```python
from build123d import *

# Parameters (mm, degrees)
F2_R     = 254
F3_DEPTH = 635
F4_R     = 127
F5_DEPTH = 1270.001


with BuildPart() as f1:
    # F0 (on Front) → F1 (revolve)
    with BuildSketch(Plane.XZ):
        with BuildLine():
            Line((-330.2, 381), (-330.2, 254))
            Line((-330.2, 254), (330.2, 254))
            Line((330.2, 254), (330.2, 381))
            Line((330.2, 381), (203.2, 381))
            Line((203.2, 381), (203.2, 889))
            Line((203.2, 889), (152.4, 889))
            ThreePointArc((152.4, 889), (0, 736.6), (-152.4, 889))
            Line((-152.4, 889), (-203.2, 889))
            Line((-203.2, 889), (-203.2, 381))
            Line((-203.2, 381), (-330.2, 381))
        make_face()
    revolve(axis=Axis((165.1, 0, 0), (1, 0, 0)))

    # F2 (on Right) → F3 (join, symmetric)
    with BuildSketch(Plane.YZ):
        Circle(F2_R)
    extrude(amount=F3_DEPTH, both=True)

    # F4 (on face) → F5 (cut, through all)
    with BuildSketch(Plane.YZ.offset(635)):
        Circle(F4_R)
    extrude(amount=-F5_DEPTH, mode=Mode.SUBTRACT)


solid = f1.part
```
Read the model definition and answer for the solid it produces. Units are mm, in the model's axes. A direction names the side the tool comes from. Give positions to 0.01 mm unless a question says otherwise; leave off trailing zeros. Order: outer loops, then holes, each group sorted by start corner. A loop starts at its lowest first (then second) coordinate and runs counter-clockwise, first axis right, second up.
(1) Find section C-C (x = -179.5). Give the vertices of the cut face in (y, z), plus the area to 3 significant figures.
(2) Find section A-A (y = 0). Give the vertices of the cut face in (x, z).
(3) For faces 4 (the flat face through (203.2, -12, -383)), 5 (the flat face through (-203.2, -12, 383)), 6 (the flat face through (-635, 53, 116)), determine the directions among +Z, -Z, +X, -X, +Y, -Y from which every point of the face is accessible in a straight line to the end or side of a thin tool.
(4) Find section D-D (x = -422). Give the vertices of the cut face in (y, z), plus the area to 3 significant figures.
(5) Straight lines are drawn through the part: L1, parallel to Z at x = 215, y = 0; L2, parallel to X at y = 242, z = -558; L3, parallel to X at y = -438, z = -658. For each, find the intervals that lie inside material, in ascending order.
(6) Given pin 1 (8 mm diameter, centred on y = -163, z = 399, fed in from -X); pin 2 (10 mm diameter, centred on x = -199.5, y = 188, fed in from +Z); pin 3 (4 mm diameter, centred on y = 222.5, z = -607, fed in from +X), each flat-ended and moving along its own axis, determine where each tip first touches the part or whether it passes through.
(7) For a pull along Z with two mould halves and no side action, classify faces 1 (the flat face through (330.2, 249, -79)), 2 (the cylindrical face through (8.89, -27.53, -123.98)), 3 (the cylindrical face through (-267.59, 231.83, -302.35)) as released by +Z, released by -Z, zero draft, split by the parting line, or undercut.
Result sheet:
1. outline: circle Ø1778 at (0, 0); hole circle Ø254 at (0, 0)
1. area: 2,430,000 mm2
2. outline: (-635, -254) - (-330.2, -254) - (-330.2, -381) - (-203.2, -381) - (-203.2, -889) - (-152.4, -889) arc R152.4 cw to (152.4, -889) - (203.2, -889) - (203.2, -381) - (330.2, -381) - (330.2, -254) - (635, -254) - (635, -127) - (-635, -127) - close; (-635, 127) - (635, 127) - (635, 254) - (330.2, 254) - (330.2, 381) - (203.2, 381) - (203.2, 889) - (152.4, 889) arc R152.4 cw to (-152.4, 889) - (-203.2, 889) - (-203.2, 381) - (-330.2, 381) - (-330.2, 254) - (-635, 254) - close
3. face 4: +X
3. face 5: -X
3. face 6: +Z, -Z, -X, +Y, -Y
4. outline: circle Ø508 at (0, 0); hole circle Ø254 at (0, 0)
4. area: 152,000 mm2
5. L1: z = -381 to -127, 127 to 381
5. L2: x = -203.2 to 203.2
5. L3: x = -203.2 to -116.25, 116.25 to 203.2
6. pin 1: stops at x = -203.2
6. pin 2: stops at z = 869.96
6. pin 3: stops at x = 203.2
7. face 1: zero draft
7. face 2: undercut
7. face 3: split by the parting line
